The model under review builds one solid part; all positions refer to its coordinate system, in mm. A direction names the side the tool comes from. Give positions to 0.01 mm unless a question says otherwise; leave off trailing zeros. Order: outer loops, then holes, each group sorted by start corner. A loop starts at its lowest first (then second) coordinate and runs counter-clockwise, first axis right, second up. Notation, with made-up numbers: (-18, -34) - (27, -34) arc R16 ccw to (27, -20) - close; hole circle Ø3 at (-34, 80.25). An arc over 180 degrees is marked (long way). Put each result on its own line as item: value.
```python
from build123d import *

# Parameters (mm, degrees)
SKETCH_1_W          = 79.3
SKETCH_1_H          = 45.76
EXTRUDE_1_DEPTH     = 4
SKETCH_2_W          = 7.8
SKETCH_2_H          = 45.76
EXTRUDE_2_DEPTH     = 7
CUT_EXTRUDE_1_REACH = 84.831
SKETCH_3_R          = 2.35
SKETCH_4_R          = 2.85
CUT_EXTRUDE_2_DEPTH = 0.5
CUT_EXTRUDE_START   = -0.5
SKETCH_5_R          = 2.85
CUT_EXTRUDE_3_DEPTH = 0.5
SKETCH_6_W          = 23.51189996
SKETCH_6_H          = 6.871263118
EXTRUDE_4_DEPTH     = 24
SKETCH_7_R          = 2.35
CUT_EXTRUDE_4_DEPTH = 58.27591125
SKETCH_8_R          = 2.85
CUT_EXTRUDE_5_DEPTH = 0.5
SKETCH_9_R          = 2.85
CUT_EXTRUDE_6_DEPTH = 0.5
FILLET_1_R          = 2
FILLET_2_R          = 2
FILLET_3_R          = 2
SKETCH_10_R         = 1.75
CUT_EXTRUDE_7_DEPTH = 4


with BuildPart() as part:
    # Эскиз1 → Бобышка-Вытянуть1 (new body)
    with BuildSketch(Plane(origin=(0, 0, 0), x_dir=(1, 0, 0), z_dir=(0, 1, 0))):
        Rectangle(SKETCH_1_W, SKETCH_1_H)
    extrude(amount=EXTRUDE_1_DEPTH)

    # Эскиз2 → Бобышка-Вытянуть2 (add)
    with BuildSketch(Plane.XZ):
        with Locations((-35.75, 0)):
            Rectangle(SKETCH_2_W, SKETCH_2_H)
    extrude(amount=EXTRUDE_2_DEPTH)

    # Эскиз3 → Вырез-Вытянуть1 (cut, up to next)
    with BuildSketch(Plane.ZY.offset(39.65), mode=Mode.PRIVATE) as cut_extrude_1_sk1:
        with Locations((0, -3.5)):
            Circle(SKETCH_3_R)
    cut_extrude_1_tool1 = extrude(cut_extrude_1_sk1.sketch, amount=-CUT_EXTRUDE_1_REACH, mode=Mode.PRIVATE) & part.part
    # Эскиз3 → Вырез-Вытянуть1 (cut, up to next)
    with BuildSketch(Plane.ZY.offset(39.65), mode=Mode.PRIVATE) as cut_extrude_1_sk2:
        with Locations((-8, -3.5)):
            Circle(SKETCH_3_R)
    cut_extrude_1_tool2 = extrude(cut_extrude_1_sk2.sketch, amount=-CUT_EXTRUDE_1_REACH, mode=Mode.PRIVATE) & part.part
    # Эскиз3 → Вырез-Вытянуть1 (cut, up to next)
    with BuildSketch(Plane.ZY.offset(39.65), mode=Mode.PRIVATE) as cut_extrude_1_sk3:
        with Locations((8, -3.5)):
            Circle(SKETCH_3_R)
    cut_extrude_1_tool3 = extrude(cut_extrude_1_sk3.sketch, amount=-CUT_EXTRUDE_1_REACH, mode=Mode.PRIVATE) & part.part
    add(cut_extrude_1_tool1.solids().sort_by_distance((-39.65, -3.5, 0))[0], mode=Mode.SUBTRACT)
    add(cut_extrude_1_tool2.solids().sort_by_distance((-39.65, -3.5, -8))[0], mode=Mode.SUBTRACT)
    add(cut_extrude_1_tool3.solids().sort_by_distance((-39.65, -3.5, 8))[0], mode=Mode.SUBTRACT)

    # Эскиз4 → Вырез-Вытянуть2 (cut)
    with BuildSketch(Plane.ZY.offset(39.65)):
        with Locations((-8, -3.5)):
            Circle(SKETCH_4_R)
        with Locations((0, -3.5)):
            Circle(SKETCH_4_R)
        with Locations((8, -3.5)):
            Circle(SKETCH_4_R)
    extrude(amount=-CUT_EXTRUDE_2_DEPTH, mode=Mode.SUBTRACT)

    # Эскиз5 → Вырез-Вытянуть3 (cut)
    with BuildSketch(Plane(origin=(-31.85, 0, 0), x_dir=(0, 0, -1), z_dir=(1, 0, 0)).offset(CUT_EXTRUDE_START)):
        with Locations(Location((-8, -3.5, 0), (0, 0, 180))):
            Circle(SKETCH_5_R)
        with Locations(Location((0, -3.5, 0), (0, 0, 180))):
            Circle(SKETCH_5_R)
        with Locations(Location((8, -3.5, 0), (0, 0, 180))):
            Circle(SKETCH_5_R)
    extrude(amount=CUT_EXTRUDE_3_DEPTH, mode=Mode.SUBTRACT)

    # Эскиз6 → Бобышка-Вытянуть4 (add)
    with BuildSketch(Plane.XZ):
        with Locations((27.89405002, 7.335631559)):
            Rectangle(SKETCH_6_W, SKETCH_6_H)
        with Locations((27.89405002, -7.335631559)):
            Rectangle(SKETCH_6_W, SKETCH_6_H)
    extrude(amount=EXTRUDE_4_DEPTH)

    # Эскиз7 → Вырез-Вытянуть4 (cut, through all)
    with BuildSketch(Plane(origin=(0, 0, -10.771263118), x_dir=(-1, 0, 0), z_dir=(0, 0, -1))):
        with Locations((-27.89405002, -20.1)):
            Circle(SKETCH_7_R)
        with Locations((-19.89405002, -20.1)):
            Circle(SKETCH_7_R)
        with Locations((-35.89405002, -20.1)):
            Circle(SKETCH_7_R)
    extrude(amount=-CUT_EXTRUDE_4_DEPTH, mode=Mode.SUBTRACT)

    # Эскиз8 → Вырез-Вытянуть5 (cut)
    with BuildSketch(Plane.XY.offset(10.771263118)):
        with Locations((19.89405002, -20.1)):
            Circle(SKETCH_8_R)
        with Locations((27.89405002, -20.1)):
            Circle(SKETCH_8_R)
        with Locations((35.89405002, -20.1)):
            Circle(SKETCH_8_R)
    extrude(amount=-CUT_EXTRUDE_5_DEPTH, mode=Mode.SUBTRACT)

    # Эскиз9 → Вырез-Вытянуть6 (cut)
    with BuildSketch(Plane(origin=(0, 0, -10.771263118), x_dir=(-1, 0, 0), z_dir=(0, 0, -1)).offset(CUT_EXTRUDE_START)):
        with Locations(Location((-35.89405002, -20.1, 0), (0, 0, 180))):
            Circle(SKETCH_9_R)
        with Locations(Location((-27.89405002, -20.1, 0), (0, 0, 180))):
            Circle(SKETCH_9_R)
        with Locations(Location((-19.89405002, -20.1, 0), (0, 0, 180))):
            Circle(SKETCH_9_R)
    extrude(amount=CUT_EXTRUDE_6_DEPTH, mode=Mode.SUBTRACT)

    # Скругление1
    fillet_1_edges = [part.edges().sort_by_distance(p)[0] for p in [
        (16.13810004, -24, -7.335631559),
        (39.65, -24, -7.335631559),
    ]]
    fillet(fillet_1_edges, radius=FILLET_1_R)

    # Скругление2
    fillet_2_edges = [part.edges().sort_by_distance(p)[0] for p in [
        (39.65, -24, 7.335631559),
        (16.13810004, -24, 7.335631559),
    ]]
    fillet(fillet_2_edges, radius=FILLET_2_R)

    # Скругление3
    fillet_3_edges = [part.edges().sort_by_distance(p)[0] for p in [
        (-35.75, -7, -22.88),
        (-35.75, -7, 22.88),
    ]]
    fillet(fillet_3_edges, radius=FILLET_3_R)

    # Эскиз10 → Вырез-Вытянуть7 (cut)
    with BuildSketch(Plane(origin=(0, 4, 0), x_dir=(1, 0, 0), z_dir=(0, 1, 0))):
        with Locations(Location((29.65, 16, 0), (0, 0, 270))):
            Circle(SKETCH_10_R)
        with Locations(Location((29.65, -16, 0), (0, 0, 270))):
            Circle(SKETCH_10_R)
        with Locations(Location((21.65, 16, 0), (0, 0, 270))):
            Circle(SKETCH_10_R)
        with Locations(Location((21.65, -16, 0), (0, 0, 270))):
            Circle(SKETCH_10_R)
        with Locations(Location((13.65, 16, 0), (0, 0, 270))):
            Circle(SKETCH_10_R)
        with Locations(Location((13.65, -16, 0), (0, 0, 270))):
            Circle(SKETCH_10_R)
        with Locations(Location((5.65, 16, 0), (0, 0, 270))):
            Circle(SKETCH_10_R)
        with Locations(Location((5.65, -16, 0), (0, 0, 270))):
            Circle(SKETCH_10_R)
        with Locations(Location((-2.35, 16, 0), (0, 0, 270))):
            Circle(SKETCH_10_R)
        with Locations(Location((-2.35, -16, 0), (0, 0, 270))):
            Circle(SKETCH_10_R)
        with Locations(Location((-10.35, 16, 0), (0, 0, 270))):
            Circle(SKETCH_10_R)
        with Locations(Location((-10.35, -16, 0), (0, 0, 270))):
            Circle(SKETCH_10_R)
        with Locations(Location((-18.35, 16, 0), (0, 0, 270))):
            Circle(SKETCH_10_R)
        with Locations(Location((-18.35, -16, 0), (0, 0, 270))):
            Circle(SKETCH_10_R)
        with Locations(Location((-26.35, 16, 0), (0, 0, 270))):
            Circle(SKETCH_10_R)
        with Locations(Location((-26.35, -16, 0), (0, 0, 270))):
            Circle(SKETCH_10_R)
    extrude(amount=-CUT_EXTRUDE_7_DEPTH, mode=Mode.SUBTRACT)


solid = part.part
```
(1) Wall thickness on L1, parallel to Z at x = 20.5, y = -2.5; L2, parallel to Z at x = 33.5, y = -20.5; L3, parallel to Z at x = -25, y = 0.5: over which ranges is each line inside the solid? List them lowest first.
The answers:
L1: -10.77 to -3.9, 3.9 to 10.77
L2: -10.27 to -3.9, 3.9 to 10.27
L3: -22.88 to -17.11, -14.89 to 14.89, 17.11 to 22.88
(2) The part is to be moulded in two halves that separate along X. For faces 4 (the cylindrical face through (37.21, -17.57, -10.52)), 5 (the cylindrical face through (39.08, -23.4, 7.38)), 6 (the flat face through (28, -9, 10.771)), 7 (the flat face through (-39.15, -1, -1)), say which applies: pulls with the +X half, pulls with the -X half, needs draft (parallel to the pull), parting line crosses it, or undercut.
The answers:
face 4: undercut
face 5: pulls with the +X half
face 6: needs draft
face 7: pulls with the -X half
(3) Clearance check with flat-ended pins moving along their axes: pin 1 Ø8 at (x, z) = (-9.5, 16) entering from -Y; pin 2 Ø1.7 at (y, z) = (-3, -8.5) entering from -X; pin 3 Ø6.5 at (x, y) = (37, -20.5) entering from -Z; pin 4 Ø4.5 at (x, z) = (-2.35, -16) entering from +Y. State where each tip first meets the part, or that it passes through.
The answers:
pin 1: y = 0
pin 2: x = 16.14
pin 3: z = -10.77
pin 4: y = 4
(4) Take a section at C-C, the plane y = -3.5. Count the separate pieces of the cut face and the enclosed holes in it, then the cut area to 3 significant figures.
The answers:
separate pieces: 6
enclosed holes: 0
area: 567 mm^2
(5) Take a section at A-A, the plane z = 8. Write out the cut boundary in (x, y), then the cut area to 3 significant figures.
The answers:
outline: (-39.65, -7) - (-31.85, -7) - (-31.85, -6.35) - (-32.35, -6.35) - (-32.35, -5.85) - (-39.15, -5.85) - (-39.15, -6.35) - (-39.65, -6.35) - close; (-39.65, -0.65) - (-39.15, -0.65) - (-39.15, -1.15) - (-32.35, -1.15) - (-32.35, -0.65) - (-31.85, -0.65) - (-31.85, 0) - (16.14, 0) - (16.14, -22) arc R2 ccw to (18.14, -24) - (37.65, -24) arc R2 ccw to (39.65, -22) - (39.65, 4) - (-39.65, 4) - close; hole circle Ø4.7 at (19.89, -20.1); hole circle Ø4.7 at (27.89, -20.1); hole circle Ø4.7 at (35.89, -20.1)
area: 845 mm^2
(6) For faces 1 (the flat face through (26, -22, -10.271)), 2 (the flat face through (-32.35, -6, -8)), 3 (the cylindrical face through (27.523, -17.274, 10.525)), list the 3-axis set-ups (+Z, -Z, +X, -X, +Y, -Y) from which the entire face can be reached by the end or side of a thin tool; tool diameter is ignored.
The answers:
face 1: -Z
face 2: none
face 3: +Z
(7) Take a section at B-B, the plane x = -2.35. Write out the cut boundary in (y, z).
The answers:
outline: (0, -22.88) - (4, -22.88) - (4, -17.75) - (0, -17.75) - close; (0, -14.25) - (4, -14.25) - (4, 14.25) - (0, 14.25) - close; (0, 17.75) - (4, 17.75) - (4, 22.88) - (0, 22.88) - close
